Build history of the part. All positions in model axes, mm. A direction names the side the tool comes from. Coordinates: 2 decimals unless noted, no trailing zeros. Order: outer loops, then holes, each group sorted by start corner. A loop starts at its lowest first (then second) coordinate and runs counter-clockwise, first axis right, second up. Notation, with made-up numbers: (-26, 15.25) - (-19, 15.25) arc R24 ccw to (-19, 35.25) - close; hole circle Ø3 at (32.5, -17). An arc over 180 degrees is marked (long way). One line per item, written item: value.
from build123d import *

# Parameters (mm, degrees)
SKETCH_1_W          = 2
SKETCH_1_H          = 120
EXTRUDE_1_DEPTH     = 2
SKETCH_3_W          = 120
SKETCH_3_H          = 20
EXTRUDE_3_DEPTH     = 15
SKETCH_4_W          = 10
SKETCH_4_H          = 11
CUT_EXTRUDE_1_DEPTH = 123.702893201
SKETCH_5_W          = 2
SKETCH_5_H          = 17
CUT_EXTRUDE_2_DEPTH = 66.238025721
SKETCH_6_W          = 15
SKETCH_6_H          = 5
EXTRUDE_4_DEPTH     = 11
SKETCH_7_R          = 0.75
CUT_EXTRUDE_3_DEPTH = 2
CUT_EXTRUDE_START   = -118
SKETCH_7_3_R        = 0.75
CUT_EXTRUDE_4_DEPTH = 2
SKETCH_8_R          = 0.8
CUT_EXTRUDE_5_DEPTH = 2


with BuildPart() as part:
    # 草图1 → 凸台-拉伸1 (new body)
    with BuildSketch(Plane(origin=(0, 0, 0), x_dir=(1, 0, 0), z_dir=(0, 1, 0))):
        Rectangle(SKETCH_1_W, SKETCH_1_H)
    extrude(amount=EXTRUDE_1_DEPTH)

    # 草图3 → 凸台-拉伸3 (add)
    with BuildSketch(Plane(origin=(1, 0, 0), x_dir=(0, 0, -1), z_dir=(1, 0, 0))):
        with Locations((0, 10)):
            Rectangle(SKETCH_3_W, SKETCH_3_H)
    extrude(amount=EXTRUDE_3_DEPTH)

    # 草图4 → 切除-拉伸1 (cut, through all)
    with BuildSketch(Plane.XY.offset(60)):
        with Locations((6, 14.5)):
            Rectangle(SKETCH_4_W, SKETCH_4_H)
    extrude(amount=-CUT_EXTRUDE_1_DEPTH, mode=Mode.SUBTRACT)

    # 草图5 → 切除-拉伸2 (cut, through all)
    with BuildSketch(Plane.XZ):
        with Locations((0, 51.5)):
            Rectangle(SKETCH_5_W, SKETCH_5_H)
        with Locations((0, -51.5)):
            Rectangle(SKETCH_5_W, SKETCH_5_H)
    extrude(amount=-CUT_EXTRUDE_2_DEPTH, mode=Mode.SUBTRACT)

    # 草图6 → 凸台-拉伸4 (add)
    with BuildSketch(Plane(origin=(0, 9, 0), x_dir=(1, 0, 0), z_dir=(0, 1, 0))):
        with Locations((8.5, -57.5)):
            Rectangle(SKETCH_6_W, SKETCH_6_H)
        with Locations((8.5, 57.5)):
            Rectangle(SKETCH_6_W, SKETCH_6_H)
    extrude(amount=EXTRUDE_4_DEPTH)

    # 草图7 → 切除-拉伸3 (cut)
    with BuildSketch(Plane(origin=(0, 0, -60), x_dir=(-1, 0, 0), z_dir=(0, 0, -1))):
        with Locations((-6, 15)):
            Circle(SKETCH_7_R)
        with Locations((-6, 5)):
            Circle(SKETCH_7_R)
    extrude(amount=-CUT_EXTRUDE_3_DEPTH, mode=Mode.SUBTRACT)

    # 草图7<3> → 切除-拉伸4 (cut)
    with BuildSketch(Plane(origin=(0, 0, -60), x_dir=(-1, 0, 0), z_dir=(0, 0, -1)).offset(CUT_EXTRUDE_START)):
        with Locations((-6, 15)):
            Circle(SKETCH_7_3_R)
        with Locations((-6, 5)):
            Circle(SKETCH_7_3_R)
    extrude(amount=-CUT_EXTRUDE_4_DEPTH, mode=Mode.SUBTRACT)

    # 草图8 → 切除-拉伸5 (cut)
    with BuildSketch(Plane(origin=(0, 20, 0), x_dir=(1, 0, 0), z_dir=(0, 1, 0))):
        with Locations(Location((13.5, -57.5, 0), (0, 0, 270))):
            Circle(SKETCH_8_R)
        with Locations(Location((13.5, 57.5, 0), (0, 0, 270))):
            Circle(SKETCH_8_R)
    extrude(amount=-CUT_EXTRUDE_5_DEPTH, mode=Mode.SUBTRACT)


solid = part.part
1. Band-saw the part on C-C, the plane y = 7.5. Give the cut face in (x, z).
Values found:
outline: (1, -60) - (16, -60) - (16, 60) - (1, 60) - close
2. Band-saw the part on B-B, the plane x = 3. Give the cut face in (y, z), and give its area (3 significant figures).
Values found:
outline: (0, -60) - (20, -60) - (20, -55) - (9, -55) - (9, 55) - (20, 55) - (20, 60) - (0, 60) - close
area: 1,190 mm2
3. Band-saw the part on A-A, the plane y = 12.25. Give the cut face in (x, z).
Values found:
outline: (1, -60) - (16, -60) - (16, 60) - (1, 60) - (1, 55) - (11, 55) - (11, -55) - (1, -55) - close
4. Probe line 1 along Y through (x, z) = (6, -59.25); line 2 along Z through (x, y) = (6.25, 15); line 3 along Z through (x, y) = (3.75, 14.5). List the from-to ranges inside material, lowest first.
Values found:
line 1: y = 0 to 4.25, 5.75 to 14.25, 15.75 to 20
line 2: z = -58 to -55, 55 to 58
line 3: z = -60 to -55, 55 to 60
5. Two-plate mould, pull along Z, no slides. Class faces 6 (the face through (8, 10, -60)), 7 (the face through (7, 0, 1)), 8 (the face through (6, 14, 55)): pulls with the +Z half, pulls with the -Z half, needs draft (parallel to the pull), parting line crosses it, or undercut.
Values found:
face 6: pulls with the -Z half
face 7: needs draft
face 8: undercut
6. 3-axis set-ups, long thin cutter, end or side, ignore diameter. For faces 1 (the face through (16, 10, 1)), 2 (the face through (0, 2, -1)), 3 (the face through (0, 1, -43)), 4 (the face through (0, 1, 43)), 5 (the face through (6, 14, -55)): which of +Z, -Z, +X, -X, +Y, -Y reach the whole face in a straight line?
Values found:
face 1: +Z, -Z, +X, +Y, -Y
face 2: +Z, -Z, -X, +Y
face 3: -Z, -X, +Y, -Y
face 4: +Z, -X, +Y, -Y
face 5: -X, +Y
7. Flat gauge pins, fed straight in: P1, Ø5, axis at x = 4.5, z = 19, coming from the +Y side; P2, Ø0.6, axis at x = 0, y = 1, coming from the +Z side; P3, Ø1.3, axis at x = 13.5, z = -57.5, coming from the +Y side. Where does each tip first touch, or does it go through?
Values found:
P1: stops at y = 9
P2: stops at z = 43
P3: stops at y = 18
